Geometry: final body of the model. Coordinates: model frame, mm. Give positions to 0.01 mm unless a question says otherwise; leave off trailing zeros. Write each loop counter-clockwise with the first axis right and the second up, starting at its lowest first coordinate (ties: lowest second). Pieces come first, ordered by that corner, then holes. Notation, with made-up numbers: (6.25, 29.5) -> (57.25, 29.5) arc R26 cw to (57.25, 55.5) -> close; hole circle Ø10 at (83.25, 78). An arc over 180 degrees is marked (long way). Use CSV: the item, a comma, the result in double quotes. Start each with the question number.
1) Section B-B (x = 130). Output: boundary loops of the cut face in (y, z), plus the area to 3 significant figures.
2) Material intervals for line 1 (X direction, y = 1.05, z = 130); line 2 (Z direction, x = -44, y = 3.15); line 3 (Z direction, x = -125.5, y = 1), sorted ascending. Write a range as [from, to].
3) Section A-A (x = 48.5). Output: boundary loops of the cut face in (y, z), plus the area to 3 significant figures.
4) Contact query for flat-ended pins moving along their axis: P1, Ø1.2, axis at y = 2, z = 131, coming from the +X side; P2, Ø2, axis at y = 2, z = 125.5, coming from the -X side; P3, Ø1.2, axis at x = -112.5, y = 1, coming from the +Z side. Output: stop coordinate, or through.
```python
from build123d import *

# Parameters (mm, degrees)
SKETCH1_W           = 340
SKETCH1_H           = 340
BOSS_EXTRUDE1_DEPTH = 4
CUT_EXTRUDE1_DEPTH  = 10
CUT_EXTRUDE2_DEPTH  = 10
CUT_EXTRUDE3_DEPTH  = 10
CUT_EXTRUDE4_DEPTH  = 10
FILLET1_R           = 2
SKETCH6_W           = 392.3816867
SKETCH6_H           = 384.263444906
SKETCH6_W_2         = 310.4
SKETCH6_H_2         = 310.4
CUT_EXTRUDE5_DEPTH  = 10


with BuildPart() as part:
    # Sketch1 → Boss-Extrude1 (new body)
    with BuildSketch(Plane(origin=(0, 0, 0), x_dir=(1, 0, 0), z_dir=(0, 1, 0))):
        Rectangle(SKETCH1_W, SKETCH1_H)
    extrude(amount=BOSS_EXTRUDE1_DEPTH)

    # Sketch2 → Cut-Extrude1 (cut)
    with BuildSketch(Plane.XZ):
        with BuildLine():
            Line((-66.986059773, -127.64), (-66.986059773, -170))
            Line((-66.986059773, -170), (-31.986059773, -170))
            Line((-31.986059773, -170), (-31.986059773, -127.64))
            ThreePointArc((-31.986059773, -127.64), (-33.450525867, -124.104466094), (-36.986059773, -122.64))
            Line((-36.986059773, -122.64), (-61.986059773, -122.64))
            ThreePointArc((-61.986059773, -122.64), (-65.521593679, -124.104466094), (-66.986059773, -127.64))
        make_face()
        with BuildLine():
            Line((-67.986059773, -170), (-66.986059773, -170))
            Line((-66.986059773, -170), (-66.986059773, -127.64))
            ThreePointArc((-66.986059773, -127.64), (-65.521593679, -124.104466094), (-61.986059773, -122.64))
            Line((-61.986059773, -122.64), (-36.986059773, -122.64))
            ThreePointArc((-36.986059773, -122.64), (-33.450525867, -124.104466094), (-31.986059773, -127.64))
            Line((-31.986059773, -127.64), (-31.986059773, -170))
            Line((-31.986059773, -170), (-30.986059773, -170))
            Line((-30.986059773, -170), (-30.986059773, -127.64))
            ThreePointArc((-30.986059773, -127.64), (-32.743419086, -123.397359313), (-36.986059773, -121.64))
            Line((-36.986059773, -121.64), (-61.986059773, -121.64))
            ThreePointArc((-61.986059773, -121.64), (-66.22870046, -123.397359313), (-67.986059773, -127.64))
            Line((-67.986059773, -127.64), (-67.986059773, -170))
        make_face()
    extrude(amount=-CUT_EXTRUDE1_DEPTH, mode=Mode.SUBTRACT)

    # Sketch3 → Cut-Extrude2 (cut)
    with BuildSketch(Plane.XZ):
        with BuildLine():
            Line((-170, 170), (-170, 100.75796452))
            Line((-170, 100.75796452), (-155.526912903, 92.401923789))
            ThreePointArc((-155.526912903, 92.401923789), (-154.803370039, 92.102222521), (-154.026912903, 92))
            Line((-154.026912903, 92), (-126.103320198, 92))
            ThreePointArc((-126.103320198, 92), (-123.981999855, 92.878679656), (-123.103320198, 95))
            Line((-123.103320198, 95), (-123.103320198, 103))
            ThreePointArc((-123.103320198, 103), (-122.224640542, 105.121320344), (-120.103320198, 106))
            Line((-120.103320198, 106), (-109.14, 106))
            ThreePointArc((-109.14, 106), (-107.018679656, 106.878679656), (-106.14, 109))
            Line((-106.14, 109), (-106.14, 148))
            Line((-106.14, 148), (-110.172231068, 170))
            Line((-110.172231068, 170), (-170, 170))
        make_face()
        with BuildLine():
            Line((-155.526912903, 92.401923789), (-170, 100.75796452))
            Line((-170, 100.75796452), (-170, 91))
            Line((-170, 91), (-154.026912903, 91))
            Line((-154.026912903, 91), (-126.103320198, 91))
            ThreePointArc((-126.103320198, 91), (-123.274893074, 92.171572875), (-122.103320198, 95))
            Line((-122.103320198, 95), (-122.103320198, 103))
            ThreePointArc((-122.103320198, 103), (-121.517533761, 104.414213562), (-120.103320198, 105))
            Line((-120.103320198, 105), (-109.14, 105))
            ThreePointArc((-109.14, 105), (-106.311572875, 106.171572875), (-105.14, 109))
            Line((-105.14, 109), (-105.14, 148.090884654))
            Line((-105.14, 148.090884654), (-105.14, 170))
            Line((-105.14, 170), (-110.172231068, 170))
            Line((-110.172231068, 170), (-106.14, 148))
            Line((-106.14, 148), (-106.14, 109))
            ThreePointArc((-106.14, 109), (-107.018679656, 106.878679656), (-109.14, 106))
            Line((-109.14, 106), (-120.103320198, 106))
            ThreePointArc((-120.103320198, 106), (-122.224640542, 105.121320344), (-123.103320198, 103))
            Line((-123.103320198, 103), (-123.103320198, 95))
            ThreePointArc((-123.103320198, 95), (-123.981999855, 92.878679656), (-126.103320198, 92))
            Line((-126.103320198, 92), (-154.026912903, 92))
            ThreePointArc((-154.026912903, 92), (-154.803370039, 92.102222521), (-155.526912903, 92.401923789))
        make_face()
    cut_extrude2 = extrude(amount=-CUT_EXTRUDE2_DEPTH, mode=Mode.SUBTRACT)

    # Mirror1: Cut-Extrude2 across plane
    add(cut_extrude2.mirror(Plane(origin=(0, 0, 0), x_dir=(0, 0, 1), z_dir=(1, 0, 0))), mode=Mode.SUBTRACT)

    # Sketch4 → Cut-Extrude3 (cut)
    with BuildSketch(Plane.XZ):
        with BuildLine():
            Line((26.206059773, -109), (26.206059773, -170))
            Line((26.206059773, -170), (72.206059773, -170))
            Line((72.206059773, -170), (72.206059773, -109))
            ThreePointArc((72.206059773, -109), (71.327380117, -106.878679656), (69.206059773, -106))
            Line((69.206059773, -106), (29.206059773, -106))
            ThreePointArc((29.206059773, -106), (27.08473943, -106.878679656), (26.206059773, -109))
        make_face()
        with BuildLine():
            Line((25.206059773, -170), (26.206059773, -170))
            Line((26.206059773, -170), (26.206059773, -109))
            ThreePointArc((26.206059773, -109), (27.08473943, -106.878679656), (29.206059773, -106))
            Line((29.206059773, -106), (69.206059773, -106))
            ThreePointArc((69.206059773, -106), (71.327380117, -106.878679656), (72.206059773, -109))
            Line((72.206059773, -109), (72.206059773, -170))
            Line((72.206059773, -170), (73.206059773, -170))
            Line((73.206059773, -170), (73.206059773, -109))
            ThreePointArc((73.206059773, -109), (72.034486898, -106.171572875), (69.206059773, -105))
            Line((69.206059773, -105), (29.206059773, -105))
            ThreePointArc((29.206059773, -105), (26.377632649, -106.171572875), (25.206059773, -109))
            Line((25.206059773, -109), (25.206059773, -170))
        make_face()
    extrude(amount=-CUT_EXTRUDE3_DEPTH, mode=Mode.SUBTRACT)

    # Sketch5 → Cut-Extrude4 (cut)
    with BuildSketch(Plane.XZ):
        Polygon((136, -170), (136, -149.5), (149.5, -149.5), (149.5, -136), (170, -136), (170, -170), align=None)
        Polygon((-170, -136), (-149.5, -136), (-149.5, -149.5), (-136, -149.5), (-136, -170), (-170, -170), align=None)
    extrude(amount=-CUT_EXTRUDE4_DEPTH, mode=Mode.SUBTRACT)

    # Fillet1
    fillet1_edges = [part.edges().sort_by_distance(p)[0] for p in [
        (136, 2, -149.5),
        (149.5, 2, -136),
        (-149.5, 2, -136),
        (-136, 2, -149.5),
    ]]
    fillet(fillet1_edges, radius=FILLET1_R)

    # Sketch6 → Cut-Extrude5 (cut)
    with BuildSketch(Plane(origin=(0, 0, 0), x_dir=(1, 0, 0), z_dir=(0, 1, 0))):
        Rectangle(SKETCH6_W, SKETCH6_H)
        Rectangle(SKETCH6_W_2, SKETCH6_H_2, mode=Mode.SUBTRACT)
    extrude(amount=CUT_EXTRUDE5_DEPTH, mode=Mode.SUBTRACT)


solid = part.part
```
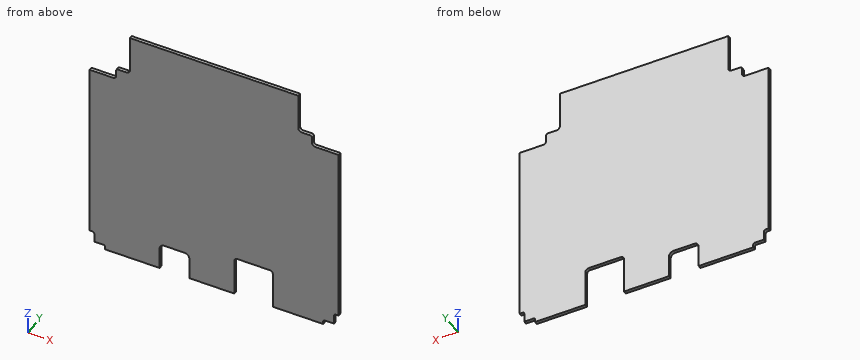
Answers follow:
1,outline,"(0, -155.2) -> (4, -155.2) -> (4, 91) -> (0, 91) -> close"
1,area,"985 mm^2"
2,line 1,"x = [-105.14, 105.14]"
2,line 2,"z = [-121.64, 155.2]"
2,line 3,"z = [-155.2, 91.05]"
3,outline,"(0, -105) -> (4, -105) -> (4, 155.2) -> (0, 155.2) -> close"
3,area,"1,040 mm^2"
4,P1,"stops at x = 105.14"
4,P2,"stops at x = -105.14"
4,P3,"stops at z = 105"
